Source: CAD feature listing. Evaluate the final solid. Frame: model axes, mm. A direction names the side the tool comes from. Give positions to 0.01 mm unless a question says otherwise; leave off trailing zeros. Write each loop counter-clockwise with the first axis right and the second up, starting at its lowest first coordinate (ties: lowest second). Pieces come first, ordered by that corner, then holes. Notation, with made-up numbers: (-5.5, 76.25) -> (13.5, 76.25) arc R21 ccw to (13.5, 100.25) -> close; hole circle Ø8 at (1.25, 5.25). An arc over 180 degrees is marked (long way). Use one line per item in the form item = value. Start each with the question number.
(1) Cut plane B-B, the plane x = -34. Output: boundary loops of the cut face in (y, z), and give its area (3 significant figures).
(2) Material intervals for line 1 along X through (y, z) = (8.25, -4.75); line 2 along Y through (x, z) = (-47, -7.75); line 3 along X through (y, z) = (12.5, -7.25), sorted ascending. Write a range as from..to.
(3) Draft query along Y for faces 1 (the face through (-10.628, 7.142, -7.405)), 2 (the face through (-51.568, 4.098, -4.678)), 3 (the face through (-1, 20, -6)), 4 (the face through (-8.84, 5.57, -7.41)). Return one class per face: pulls with the +Y half, pulls with the -Y half, needs draft (parallel to the pull), parting line crosses it, or undercut.
(4) Set-up query: faces 5 (the face through (4, 10, -9.028)), 6 (the face through (-38, 8.083, -4)), 7 (the face through (-8.84, 5.57, -0.61)), 8 (the face through (5.03, 9.29, -3.66)). Return all of +Z, -Z, +X, -X, +Y, -Y with unobstructed straight access to the full face (end or side cutting, diameter ignored); none if empty.
(5) First-contact query: P1, Ø5, axis at y = 18, z = -5.5, coming from the -X side; P2, Ø3, axis at x = -39.5, z = -1.5, coming from the +Y side; P3, Ø1.3, axis at x = -7.35, y = 2.96, coming from the +Z side. Flat tips, straight axial feed; report the tip coordinate or a pass-through.
(6) Cut plane A-A, the plane y = 17. Output: boundary loops of the cut face in (x, z), and give its area (3 significant figures).
from build123d import *

# Parameters (mm, degrees)
SKETCH1_W                 = 20
SKETCH1_H                 = 10
BOSS_EXTRUDE1_DEPTH       = 20
SKETCH2_R                 = 2.5
CUT_EXTRUDE1_DEPTH        = 26.836409614
CUT_EXTRUDE2_DEPTH        = 27.191969955
SKETCH5_R                 = 1.95
CUT_EXTRUDE5_DEPTH        = 21.021203074
M2X0_4_TAPPED_HOLE1_D     = 1.6
M2X0_4_TAPPED_HOLE1_DEPTH = 6
M2X0_4_TAPPED_HOLE1_TIP   = 0.480688495
M2X0_4_TAPPED_HOLE2_D     = 1.6
M2X0_4_TAPPED_HOLE2_DEPTH = 6
M2X0_4_TAPPED_HOLE2_TIP   = 0.480688495
SKETCH14_W                = 10
SKETCH14_H                = 8.082903769
BOSS_EXTRUDE3_DEPTH       = 50
CUT_EXTRUDE7_REACH        = 67.371
SKETCH15_R                = 3
SKETCH16_R                = 1
CUT_EXTRUDE8_DEPTH        = 68.45300722
SKETCH18_R                = 0.5
CUT_EXTRUDE9_DEPTH        = 3


with BuildPart() as part:
    # Sketch1 → Boss-Extrude1 (new body)
    with BuildSketch(Plane(origin=(0, 0, 0), x_dir=(1, 0, 0), z_dir=(0, 1, 0))):
        with Locations((-3.638888889, 4.027777778)):
            Rectangle(SKETCH1_W, SKETCH1_H)
    extrude(amount=BOSS_EXTRUDE1_DEPTH)

    # Sketch2 → Cut-Extrude1 (cut, through all)
    with BuildSketch(Plane(origin=(0, 20, 0), x_dir=(1, 0, 0), z_dir=(0, 1, 0))):
        with Locations(Location((1.361111111, 4.027777778, 0), (0, 0, 270))):
            Circle(SKETCH2_R)
        Polygon((1.495085707, -0.972222222), (1.361111111, -0.472222222), (1.227136515, -0.972222222), align=None)
        Polygon((1.361111111, 8.527777778), (1.227136515, 9.027777778), (1.495085707, 9.027777778), align=None)
    extrude(amount=-CUT_EXTRUDE1_DEPTH, mode=Mode.SUBTRACT)

    # Sketch3 → Cut-Extrude2 (cut, through all)
    with BuildSketch(Plane.XY.offset(0.972222222)):
        Polygon((-13.638888889, 20), (-3.638888889, 20), (-3.638888889, 13.856406461), (-10.489369836, 9.901279442), (-8.200869836, 5.937481169), (-9.499907942, 5.187481169), (-11.788407942, 9.151279442), (-13.638888889, 8.082903769), align=None)
    extrude(amount=-CUT_EXTRUDE2_DEPTH, mode=Mode.SUBTRACT)

    # Sketch5 → Cut-Extrude5 (cut, through all)
    with BuildSketch(Plane(origin=(-6.909722222, 11.967989955, 0), x_dir=(0.8660254037844415, 0.49999999999999534, 0), z_dir=(-0.49999999999999534, 0.8660254037844415, 0))):
        with Locations(Location((-4.883421027, 4.027777778, 0), (0, 0, 180))):
            Circle(SKETCH5_R)
    extrude(amount=-CUT_EXTRUDE5_DEPTH, mode=Mode.SUBTRACT)

    # M2x0.4 Tapped Hole1
    with Locations(Plane(origin=(6.361111111, 0, 0), x_dir=(0, 0, -1), z_dir=(1, 0, 0))):
        with Locations((4.027777778, 10)):
            Hole(M2X0_4_TAPPED_HOLE1_D / 2, depth=M2X0_4_TAPPED_HOLE1_DEPTH)
            with Locations((0, 0, -(M2X0_4_TAPPED_HOLE1_DEPTH + M2X0_4_TAPPED_HOLE1_TIP / 2))):  # 118° drill point
                Cone(0, M2X0_4_TAPPED_HOLE1_D / 2, M2X0_4_TAPPED_HOLE1_TIP, mode=Mode.SUBTRACT)

    # M2x0.4 Tapped Hole2
    with Locations(Plane.XY.offset(0.972222222)):
        with Locations((-7.350388889, 2.964404957)):
            Hole(M2X0_4_TAPPED_HOLE2_D / 2, depth=M2X0_4_TAPPED_HOLE2_DEPTH)
            with Locations((0, 0, -(M2X0_4_TAPPED_HOLE2_DEPTH + M2X0_4_TAPPED_HOLE2_TIP / 2))):  # 118° drill point
                Cone(0, M2X0_4_TAPPED_HOLE2_D / 2, M2X0_4_TAPPED_HOLE2_TIP, mode=Mode.SUBTRACT)

    # Sketch14 → Boss-Extrude3 (add)
    with BuildSketch(Plane.ZY.offset(13.638888889)):
        with Locations((-4.027777778, 4.041451884)):
            Rectangle(SKETCH14_W, SKETCH14_H)
    extrude(amount=BOSS_EXTRUDE3_DEPTH)

    # Sketch15 → Cut-Extrude7 (cut, up to next)
    with BuildSketch(Plane(origin=(0, 8.082903769, 0), x_dir=(1, 0, 0), z_dir=(0, 1, 0)), mode=Mode.PRIVATE) as cut_extrude7_sk1:
        with Locations(Location((-48.638888889, 4.027777778, 0), (0, 0, 270))):
            Circle(SKETCH15_R)
    cut_extrude7_tool1 = extrude(cut_extrude7_sk1.sketch, amount=-CUT_EXTRUDE7_REACH, mode=Mode.PRIVATE) & part.part
    # Sketch15 → Cut-Extrude7 (cut, up to next)
    with BuildSketch(Plane(origin=(0, 8.082903769, 0), x_dir=(1, 0, 0), z_dir=(0, 1, 0)), mode=Mode.PRIVATE) as cut_extrude7_sk2:
        with Locations(Location((-23.638888889, 4.027777778, 0), (0, 0, 270))):
            Circle(SKETCH15_R)
    cut_extrude7_tool2 = extrude(cut_extrude7_sk2.sketch, amount=-CUT_EXTRUDE7_REACH, mode=Mode.PRIVATE) & part.part
    add(cut_extrude7_tool1.solids().sort_by_distance((-48.638889, 8.082904, -4.027778))[0], mode=Mode.SUBTRACT)
    add(cut_extrude7_tool2.solids().sort_by_distance((-23.638889, 8.082904, -4.027778))[0], mode=Mode.SUBTRACT)

    # Sketch16 → Cut-Extrude8 (cut, through all)
    with BuildSketch(Plane.XY.offset(0.972222222)):
        with Locations((-61.638888889, 4)):
            Circle(SKETCH16_R)
        with Locations((-29.638888889, 4)):
            Circle(SKETCH16_R)
    extrude(amount=-CUT_EXTRUDE8_DEPTH, mode=Mode.SUBTRACT)

    # Sketch18 → Cut-Extrude9 (cut)
    with BuildSketch(Plane.XY.offset(0.972222222)):
        with Locations((-7.638888889, 8)):
            Circle(SKETCH18_R)
    extrude(amount=-CUT_EXTRUDE9_DEPTH, mode=Mode.SUBTRACT)


solid = part.part
Geometry says:
q1.outline = (0, -9.03) -> (8.08, -9.03) -> (8.08, 0.97) -> (0, 0.97) -> close
q1.area = 80.8 mm^2
q2.line_1 = -13.35..-12.49, -8.31..-1.03, 3.75..6.36
q2.line_2 = 0..8.08
q2.line_3 = -5.99..6.36
q3.face_1 = undercut
q3.face_2 = needs draft
q3.face_3 = pulls with the +Y half
q3.face_4 = undercut
q4.face_5 = -Z, +X, -X, +Y, -Y
q4.face_6 = +Z, -Z, -X, +Y
q4.face_7 = +Z, -Z
q4.face_8 = +X
q5.P1 = -3.64
q5.P2 = 8.08
q5.P3 = -5.87
q6.outline = (-3.64, -9.03) -> (1.23, -9.03) -> (1.36, -8.53) -> (1.5, -9.03) -> (6.36, -9.03) -> (6.36, 0.97) -> (1.5, 0.97) -> (1.36, 0.47) -> (1.23, 0.97) -> (-3.64, 0.97) -> close; hole circle Ø5 at (1.36, -4.03)
q6.area = 80.2 mm^2
